from build123d import *

# Parameters (mm, degrees)
SKETCH1_R           = 1.1
BOSS_EXTRUDE1_DEPTH = 3
SKETCH4_R           = 1.1
CUT_EXTRUDE2_DEPTH  = 70.014491232
SKETCH5_R           = 7.5
CUT_EXTRUDE3_DEPTH  = 70.014491232


with BuildPart() as part:
    # Sketch1 → Boss-Extrude1 (new body)
    with BuildSketch(Plane.XY):
        Polygon((-55, -20), (-25, -20), (-25, -23), (-15, -23), (-15, -20), (15, -20), (15, -23), (25, -23), (25, -20), (55, -20), (55, -23), (65, -23), (65, 23), (55, 23), (55, 20), (25, 20), (25, 23), (15, 23), (15, 20), (-15, 20), (-15, 23), (-25, 23), (-25, 20), (-55, 20), (-55, 23), (-65, 23), (-65, -23), (-55, -23), align=None)
        with Locations((32.75, 5.75)):
            Circle(SKETCH1_R, mode=Mode.SUBTRACT)
        with Locations((53.25, 5.75)):
            Circle(SKETCH1_R, mode=Mode.SUBTRACT)
        with Locations((53.25, -7.75)):
            Circle(SKETCH1_R, mode=Mode.SUBTRACT)
        with Locations((32.75, -7.75)):
            Circle(SKETCH1_R, mode=Mode.SUBTRACT)
    extrude(amount=BOSS_EXTRUDE1_DEPTH)

    # Sketch4 → Cut-Extrude2 (cut, through all)
    with BuildSketch(Plane.XY.offset(3)):
        with Locations((-20.5, 8)):
            Circle(SKETCH4_R)
        with Locations((-20.5, -8)):
            Circle(SKETCH4_R)
        with Locations((20.5, 8)):
            Circle(SKETCH4_R)
        with Locations((20.5, -8)):
            Circle(SKETCH4_R)
        with BuildLine():
            Line((-13, 8.1), (13, 8.1))
            ThreePointArc((13, 8.1), (21.1, 0), (13, -8.1))
            Line((13, -8.1), (-13, -8.1))
            ThreePointArc((-13, -8.1), (-21.1, 0), (-13, 8.1))
        make_face()
    extrude(amount=-CUT_EXTRUDE2_DEPTH, mode=Mode.SUBTRACT)

    # Sketch5 → Cut-Extrude3 (cut, through all)
    with BuildSketch(Plane.XY.offset(3)):
        with Locations((43, 0)):
            Circle(SKETCH5_R)
    extrude(amount=-CUT_EXTRUDE3_DEPTH, mode=Mode.SUBTRACT)


solid = part.part
CAD build for the part. Positions are in the model's coordinates, mm. A direction names the side the tool comes from. Give positions to 0.01 mm unless a question says otherwise; leave off trailing zeros. Loops run counter-clockwise (first coordinate to the right, second up) from the corner with the lowest first, then second, coordinate; pieces in that order, holes last. Notation, with made-up numbers: M 65,14 L 104,14 A25 cw 104,52 Z; hole C 1.25,72.25 d1. An arc over 180 degrees is marked long. One line per question, with ' | ' between items. Start each with the question number.
1. Saw through at A-A on y = 0. Give the cut face in (x, z), plus the area to 3 significant figures.
2. 3-axis set-ups, long thin cutter, end or side, ignore diameter. For faces 1 (the face through (15, -21, 1)), 2 (the face through (-40, 20, 1)), 3 (the face through (-21.6, 8, 1.5)): which of +Z, -Z, +X, -X, +Y, -Y reach the whole face in a straight line?
3. Two-plate mould, pull along X, no slides. Class faces 4 (the face through (21.1, 0.18, 1.52)), 5 (the face through (40, -20, 1)), 6 (the face through (-60, 23, 1)), 7 (the face through (-65, 0, 1)): pulls with the +X half, pulls with the -X half, needs draft (parallel to the pull), parting line crosses it, or undercut.
4. Probe L1, parallel to Y at x = 53.25, z = 2.3; L2, parallel to X at y = 5, z = 0.4; L3, parallel to X at y = 5.5, z = 1.15. List the from-to ranges inside material, lowest first. Write a range as from..to.
5. Saw through at B-B on x = 45.5. Give the cut face in (y, z).
6. Saw through at C-C on x = -49. Give the cut face in (y, z), plus the area to 3 significant figures.
7. Flat gauge pins, fed straight in: pin 1 (1.5 mm diameter, centred on x = 34.5, z = 2.5, fed in from -Y); pin 2 (3.5 mm diameter, centred on x = -20.5, y = 8, fed in from -Z); pin 3 (2 mm diameter, centred on x = 32.75, y = 5.75, fed in from -Z). Where does each tip first touch, or does it go through?
8. Saw through at D-D on z = 0.85. State how many separate pieces and enclosed holes the cut face has, plus the area to 3 significant figures.
Result sheet:
1) outline: M -65,0 L -21.1,0 L -21.1,3 L -65,3 Z; M 21.1,0 L 35.5,0 L 35.5,3 L 21.1,3 Z; M 50.5,0 L 65,0 L 65,3 L 50.5,3 Z | area: 218 mm^2
2) face 1: +Z, -Z, -Y | face 2: +Z, -Z, +Y | face 3: +Z, -Z
3) face 4: undercut | face 5: undercut | face 6: needs draft | face 7: pulls with the -X half
4) L1: y = -20..-8.85, -6.65..4.65, 6.85..20 | L2: x = -65..-19.37, 19.37..31.95, 33.55..37.41, 48.59..52.45, 54.05..65 | L3: x = -65..-18.95, 18.95..31.68, 33.82..37.9, 48.1..52.18, 54.32..65
5) outline: M -20,0 L -7.07,0 L -7.07,3 L -20,3 Z; M 7.07,0 L 20,0 L 20,3 L 7.07,3 Z
6) outline: M -20,0 L 20,0 L 20,3 L -20,3 Z | area: 120 mm^2
7) pin 1: stops at y = -20 | pin 2: stops at z = 0 | pin 3: passes through
8) separate pieces: 1 | enclosed holes: 10 | area: 4,610 mm^2
